Work out the finished part from the listing and answer in its coordinate system (mm). Face numbers are marked on the shaded views. A direction names the side the tool comes from. Round coordinates to 2 decimals unless told otherwise and drop trailing zeros. Order: outer loops, then holes, each group sorted by start corner. A loop starts at its lowest first (then second) coordinate and runs counter-clockwise, first axis right, second up. Notation, with made-up numbers: (89.5, 43.25) - (108.5, 43.25) arc R16 ccw to (108.5, 56.25) - close; hole circle Ø7 at (-19, 56). An arc over 180 degrees is marked (long way). Answer in a Markdown table with one row per item.
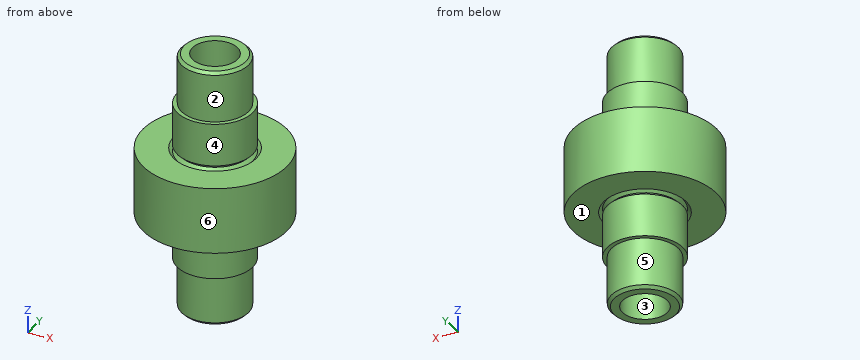
from build123d import *

# Parameters (mm, degrees)
SKETCH_2_R          = 1.5
CUT_EXTRUDE_1_DEPTH = 36.114099732
SKETCH_4_R          = 14
SKETCH_4_R_2        = 12.75
CUT_EXTRUDE_4_DEPTH = 36.114099732
CUT_EXTRUDE_5_DEPTH = 35.148572445
SKETCH_6_R          = 4
CUT_EXTRUDE_6_DEPTH = 50.594001653
SKETCH_7_R          = 12.75
SKETCH_7_R_2        = 6.7
EXTRUDE_1_DEPTH     = 11.8
CHAMFER_1_SIZE      = 0.5


with BuildPart() as part:
    # 草图1 → 旋转1 (revolve)
    with BuildSketch(Plane(origin=(0, 0, 0), x_dir=(0, 0, -1), z_dir=(1, 0, 0)), mode=Mode.PRIVATE) as revolve_1_sk:
        Polygon((-23.1, 0), (-23.1, 5.95), (-14.1, 5.95), (-14.1, 6.7), (-5.9, 6.7), (-5.9, 14), (5.9, 14), (5.9, 6.7), (14.1, 6.7), (14.1, 5.95), (23.1, 5.95), (23.1, 0), align=None)
    revolve(revolve_1_sk.sketch.rotate(Axis((0, 0, 23.1), (0, 0, -1)), 180), axis=Axis((0, 0, 23.1), (0, 0, -1)))

    # 草图2 → 切除-拉伸1 (cut, through all)
    with BuildSketch(Plane.XY.offset(5.9)):
        with Locations((0, 10.5)):
            Circle(SKETCH_2_R)
        with Locations((10.5, 0)):
            Circle(SKETCH_2_R)
        with Locations((0, -10.5)):
            Circle(SKETCH_2_R)
        with Locations((-10.5, 0)):
            Circle(SKETCH_2_R)
    extrude(amount=-CUT_EXTRUDE_1_DEPTH, mode=Mode.SUBTRACT)

    # 草图4 → 切除-拉伸4 (cut, through all)
    with BuildSketch(Plane(origin=(0, 0, -5.9), x_dir=(-1, 0, 0), z_dir=(0, 0, -1))):
        Circle(SKETCH_4_R)
        Circle(SKETCH_4_R_2, mode=Mode.SUBTRACT)
    extrude(amount=-CUT_EXTRUDE_4_DEPTH, mode=Mode.SUBTRACT)

    # 草图5 → 切除-拉伸5 (cut, through all)
    with BuildSketch(Plane(origin=(0, 0, -5.9), x_dir=(-1, 0, 0), z_dir=(0, 0, -1))):
        with BuildLine():
            Line((-9.26871571, 3.618136135), (-8.331955809, 3.252462513))
            ThreePointArc((-8.331955809, 3.252462513), (-7.618330669, 3.247249598), (-7.082950618, 3.719114215))
            ThreePointArc((-7.082950618, 3.719114215), (-5.656854249, 5.656854249), (-3.719114215, 7.082950618))
            ThreePointArc((-3.719114215, 7.082950618), (-3.247249598, 7.618330669), (-3.252462513, 8.331955809))
            Line((-3.252462513, 8.331955809), (-3.618136135, 9.26871571))
            ThreePointArc((-3.618136135, 9.26871571), (-4.194460373, 9.839863314), (-5.004644825, 9.795587281))
            ThreePointArc((-5.004644825, 9.795587281), (-7.778174593, 7.778174593), (-9.795587281, 5.004644825))
            ThreePointArc((-9.795587281, 5.004644825), (-9.839863314, 4.194460373), (-9.26871571, 3.618136135))
        make_face()
        with BuildLine():
            Line((3.618136135, 9.26871571), (3.252462513, 8.331955809))
            ThreePointArc((3.252462513, 8.331955809), (3.247249598, 7.618330669), (3.719114215, 7.082950618))
            ThreePointArc((3.719114215, 7.082950618), (5.656854249, 5.656854249), (7.082950618, 3.719114215))
            ThreePointArc((7.082950618, 3.719114215), (7.618330669, 3.247249598), (8.331955809, 3.252462513))
            Line((8.331955809, 3.252462513), (9.26871571, 3.618136135))
            ThreePointArc((9.26871571, 3.618136135), (9.839863314, 4.194460373), (9.795587281, 5.004644825))
            ThreePointArc((9.795587281, 5.004644825), (7.778174593, 7.778174593), (5.004644825, 9.795587281))
            ThreePointArc((5.004644825, 9.795587281), (4.194460373, 9.839863314), (3.618136135, 9.26871571))
        make_face()
        with BuildLine():
            Line((9.26871571, -3.618136135), (8.331955809, -3.252462513))
            ThreePointArc((8.331955809, -3.252462513), (7.618330669, -3.247249598), (7.082950618, -3.719114215))
            ThreePointArc((7.082950618, -3.719114215), (5.656854249, -5.656854249), (3.719114215, -7.082950618))
            ThreePointArc((3.719114215, -7.082950618), (3.247249598, -7.618330669), (3.252462513, -8.331955809))
            Line((3.252462513, -8.331955809), (3.618136135, -9.26871571))
            ThreePointArc((3.618136135, -9.26871571), (4.194460373, -9.839863314), (5.004644825, -9.795587281))
            ThreePointArc((5.004644825, -9.795587281), (7.778174593, -7.778174593), (9.795587281, -5.004644825))
            ThreePointArc((9.795587281, -5.004644825), (9.839863314, -4.194460373), (9.26871571, -3.618136135))
        make_face()
        with BuildLine():
            Line((-3.618136135, -9.26871571), (-3.252462513, -8.331955809))
            ThreePointArc((-3.252462513, -8.331955809), (-3.247249598, -7.618330669), (-3.719114215, -7.082950618))
            ThreePointArc((-3.719114215, -7.082950618), (-5.656854249, -5.656854249), (-7.082950618, -3.719114215))
            ThreePointArc((-7.082950618, -3.719114215), (-7.618330669, -3.247249598), (-8.331955809, -3.252462513))
            Line((-8.331955809, -3.252462513), (-9.26871571, -3.618136135))
            ThreePointArc((-9.26871571, -3.618136135), (-9.839863314, -4.194460373), (-9.795587281, -5.004644825))
            ThreePointArc((-9.795587281, -5.004644825), (-7.778174593, -7.778174593), (-5.004644825, -9.795587281))
            ThreePointArc((-5.004644825, -9.795587281), (-4.194460373, -9.839863314), (-3.618136135, -9.26871571))
        make_face()
    extrude(amount=-CUT_EXTRUDE_5_DEPTH, mode=Mode.SUBTRACT)

    # 草图6 → 切除-拉伸6 (cut, through all)
    with BuildSketch(Plane(origin=(0, 0, -23.1), x_dir=(-1, 0, 0), z_dir=(0, 0, -1))):
        Circle(SKETCH_6_R)
    extrude(amount=-CUT_EXTRUDE_6_DEPTH, mode=Mode.SUBTRACT)

    # 草图7 → 凸台-拉伸1 (add)
    with BuildSketch(Plane(origin=(0, 0, -5.9), x_dir=(-1, 0, 0), z_dir=(0, 0, -1))):
        Circle(SKETCH_7_R)
        with Locations(Location((0, 0, 0), (0, 0, 270))):
            Circle(SKETCH_7_R_2, mode=Mode.SUBTRACT)
    extrude(amount=-EXTRUDE_1_DEPTH)

    # 草图8 → 切除-旋转1 (revolve, cut)
    with BuildSketch(Plane(origin=(0, 0, 0), x_dir=(0, 0, -1), z_dir=(1, 0, 0)), mode=Mode.PRIVATE) as cut_revolve_1_sk:
        Polygon((-6.502145005, 6.7), (-5.9, 6.093231234), (-5.294771168, 6.7), (-5.9, 7.303692806), align=None)
        Polygon((6.502145005, 6.7), (5.9, 7.303692806), (5.294771168, 6.7), (5.9, 6.093231234), align=None)
    revolve(cut_revolve_1_sk.sketch.rotate(Axis((0, 0, 0), (0, 0, -1)), 90), axis=Axis((0, 0, 0), (0, 0, -1)), mode=Mode.SUBTRACT)

    # 倒角1
    chamfer_1_edges = [part.edges().sort_by_distance(p)[0] for p in [
        (0, 5.95, -23.1),
        (0, 5.95, 23.1),
    ]]
    chamfer(chamfer_1_edges, length=CHAMFER_1_SIZE)


solid = part.part
1) Which of the six approach directions +Z, -Z, +X, -X, +Y, -Y give full straight-line access (tool end or side, diameter ignored) to the marked faces 4, 5 and 6?
Filled in:
| item | result |
|---|---|
| face 4 | +Z |
| face 5 | -Z |
| face 6 | +Z, -Z |
2) Find the intervals of material crossed by probe 1 along X at (y, z) = (-0.25, -18); probe 2 along Z at (x, y) = (-6, -2.25); probe 3 along Y at (x, z) = (0, -2), in increasing order. Write a range as from..to.
Filled in:
| item | result |
|---|---|
| probe 1 | x = -5.94..-3.99, 3.99..5.94 |
| probe 2 | z = -14.1..-6.21, -5.59..5.59, 6.21..14.1 |
| probe 3 | y = -12.75..-4, 4..12.75 |
3) Each of these flat-tipped pins is pushed along its axis until it touches: pin 1 (12 mm diameter, centred on y = -8.5, z = 3.5, fed in from -X); pin 2 (13 mm diameter, centred on x = 5.5, y = 0, fed in from +Z); pin 3 (1.5 mm diameter, centred on x = -8, y = -2, fed in from +Z); pin 4 (3 mm diameter, centred on x = 8, z = -2, fed in from +Y). Where does it stop, or does it pass through?
Filled in:
| item | result |
|---|---|
| pin 1 | stops at x = -12.5 |
| pin 2 | stops at z = 23.1 |
| pin 3 | stops at z = 5.9 |
| pin 4 | stops at y = 10.97 |
4) Find section A-A, the plane z = -4. Give the vertices of the cut face in (x, y).
Filled in:
| item | result |
|---|---|
| outline | circle Ø25.5 at (0, 0); hole circle Ø8 at (0, 0) |
5) Find section B-B, the plane z = -18.5. Give the vertices of the cut face in (x, y), then the cut area to 3 significant figures.
Filled in:
| item | result |
|---|---|
| outline | circle Ø11.9 at (0, 0); hole circle Ø8 at (0, 0) |
| area | 61.0 mm^2 |
6) The mould has two halves that part along Y. Classify the marked faces 1, 2 and 3: released by +Y, released by -Y, zero draft, split by the parting line, or undercut.
Filled in:
| item | result |
|---|---|
| face 1 | zero draft |
| face 2 | split by the parting line |
| face 3 | undercut |
7) Find section C-C, the plane x = -10.25. Give the vertices of the cut face in (y, z).
Filled in:
| item | result |
|---|---|
| outline | (-7.58, -5.9) - (7.58, -5.9) - (7.58, 5.9) - (-7.58, 5.9) - close |
